Verification items for the finished model (mm, model axes). Face numbers are marked on the shaded views. A direction names the side the tool comes from. Give positions to 0.01 mm unless a question says otherwise; leave off trailing zeros. Write each loop counter-clockwise with the first axis right and the second up, starting at its lowest first coordinate (ties: lowest second). Pieces come first, ordered by that corner, then holes.
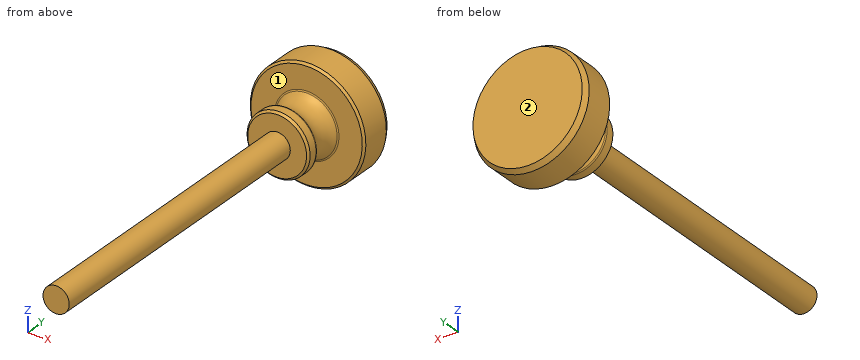
from build123d import *

# Parameters (mm, degrees)
SKETCH1_W      = 12.5
SKETCH1_H      = 300
CHAMFER1_SIZE  = 3
CHAMFER1_SIZE2 = 5.196152423
CHAMFER2_SIZE  = 2
CHAMFER3_SIZE  = 2
FILLET1_R      = 2
FILLET2_R      = 2
SCALE1_SCALE   = 0.1


with BuildPart() as part:
    # Sketch1 → Revolve1 (revolve)
    with BuildSketch(Plane.XY, mode=Mode.PRIVATE) as revolve1_sk:
        with Locations((6.25, -48.713790357)):
            Rectangle(SKETCH1_W, SKETCH1_H)
    revolve(revolve1_sk.sketch.rotate(Axis((0, 0, 0), (0, 1, 0)), 90), axis=Axis((0, 0, 0), (0, 1, 0)))

    # Sketch2 → Revolve2 (revolve)
    with BuildSketch(Plane.XY, mode=Mode.PRIVATE) as revolve2_sk:
        with BuildLine():
            Line((0, 101.286209643), (12.5, 101.286209643))
            Line((12.5, 101.286209643), (30, 101.286209643))
            Line((30, 101.286209643), (30, 112.044433041))
            ThreePointArc((30, 112.044433041), (23.556624576, 126.665321342), (30, 141.286209643))
            Line((30, 141.286209643), (55, 141.286209643))
            Line((55, 141.286209643), (55, 176.286209643))
            Line((55, 176.286209643), (0, 176.286209643))
            Line((0, 176.286209643), (0, 101.286209643))
        make_face()
    revolve(revolve2_sk.sketch.rotate(Axis((0, 0, 0), (0, 1, 0)), 90), axis=Axis((0, 0, 0), (0, 1, 0)))

    # Chamfer1
    chamfer1_edges = [part.edges().sort_by_distance(p)[0] for p in [
        (0, 176.286209643, 55),
    ]]
    chamfer1_side = [part.faces().sort_by_distance(p)[0] for p in [
        (0, 176.286209643, 0),
    ]]
    chamfer(chamfer1_edges, length=CHAMFER1_SIZE, length2=CHAMFER1_SIZE2, reference=chamfer1_side[0])

    # Chamfer2
    chamfer2_edges = [part.edges().sort_by_distance(p)[0] for p in [
        (0, 141.286209643, 55),
    ]]
    chamfer(chamfer2_edges, length=CHAMFER2_SIZE)

    # Chamfer3
    chamfer3_edges = [part.edges().sort_by_distance(p)[0] for p in [
        (0, 101.286209643, 30),
    ]]
    chamfer(chamfer3_edges, length=CHAMFER3_SIZE)

    # Fillet1
    fillet1_edges = [part.edges().sort_by_distance(p)[0] for p in [
        (0, 112.044433041, 30),
    ]]
    fillet(fillet1_edges, radius=FILLET1_R)

    # Fillet2
    fillet2_edges = [part.edges().sort_by_distance(p)[0] for p in [
        (0, 141.286209643, 30),
    ]]
    fillet(fillet2_edges, radius=FILLET2_R)


with BuildPart() as part_1:
    # Scale1: scaled about (0, 98.653209901, -1.6e-08)
    add(part.part.scale(SCALE1_SCALE).moved(Location((0, 88.787888911, -1.4e-08))))


solid = part_1.part
Item 1: Scan lines: line 1 along Y through (x, z) = (4, -2.75); line 2 along Y through (x, z) = (-2, -1); line 3 along Z through (x, y) = (-0.25, 91). Record each from-to range of solid material in increasing order.
Answer key:
line 1: y = 102.92 to 106.42
line 2: y = 98.92 to 106.42
line 3: z = -1.22 to 1.22
Item 2: Sectioned sample at B-B on y = 102. Record the cut outline in (x, z), then the cut area to 3 significant figures.
Answer key:
outline: circle Ø4.86 at (0, 0)
area: 18.6 mm2
Item 3: Sectioned sample at A-A on y = 89.5. Record the cut outline in (x, z), then the cut area to 3 significant figures.
Answer key:
outline: circle Ø2.5 at (0, 0)
area: 4.91 mm2
Item 4: Depth check by flat-ended pin: pin 1 (4 mm diameter, centred on y = 96.5, z = 2.5, fed in from -X); pin 2 (3 mm diameter, centred on y = 101, z = -1, fed in from +X); pin 3 (6 mm diameter, centred on x = -1.5, y = 87, fed in from +Z). Enter the tip coordinate at first touch or a pass-through.
Answer key:
pin 1: stops at x = -1.15
pin 2: stops at x = 3
pin 3: stops at z = 1.25
Item 5: Set-up check for the marked faces 1 and 2: record each of +Z, -Z, +X, -X, +Y, -Y from which the full face is reachable in a straight line by a thin tool's end or side.
Answer key:
face 1: -Y
face 2: +Z, -Z, +X, -X, +Y
